Can you work these out from the model? Positions are in its coordinate system, mm. A direction names the side the tool comes from. Give positions to 0.01 mm unless a question says otherwise; leave off trailing zeros. Order: outer loops, then holes, each group sorted by start corner. A loop starts at its lowest first (then second) coordinate and runs counter-clockwise, first axis right, second up. Notation, with made-up numbers: (3, -17) - (29, -17) arc R18 cw to (29, -10) - close; hole circle Ø3 at (-33.75, 59.5). An arc over 180 degrees is marked (long way). Return JSON: item names as keys, results as strings.
```python
from build123d import *

# Parameters (mm, degrees)
SALIENTE_EXTRUIR1_DEPTH = 20
CORTAR_EXTRUIR1_REACH   = 24.289
CROQUIS2_R              = 3.75
SALIENTE_EXTRUIR2_START = -9
CROQUIS3_R              = 3.75
SALIENTE_EXTRUIR2_DEPTH = 9
CROQUIS4_R              = 4.765
SALIENTE_EXTRUIR3_DEPTH = 70
CROQUIS5_R              = 13.287682266
SALIENTE_EXTRUIR4_DEPTH = 4.5


with BuildPart() as part:
    # Croquis1 → Saliente-Extruir1 (new body)
    with BuildSketch(Plane.XY):
        Polygon((-8.75, 2.25), (8.75, 2.25), (4.25, -2.25), (-4.25, -2.25), align=None)
    extrude(amount=SALIENTE_EXTRUIR1_DEPTH)

    # Croquis2 → Cortar-Extruir1 (cut, up to next)
    with BuildSketch(Plane(origin=(0, 2.25, 0), x_dir=(1, 0, 0), z_dir=(0, 1, 0)), mode=Mode.PRIVATE) as cortar_extruir1_sk1:
        with Locations(Location((0, -10, 0), (0, 0, 270))):
            Circle(CROQUIS2_R)
    cortar_extruir1_tool1 = extrude(cortar_extruir1_sk1.sketch, amount=-CORTAR_EXTRUIR1_REACH, mode=Mode.PRIVATE) & part.part
    add(cortar_extruir1_tool1.solids().sort_by_distance((0, 2.25, 10))[0], mode=Mode.SUBTRACT)

    # Croquis3 → Saliente-Extruir2 (add)
    with BuildSketch(Plane.XZ.offset(2.25).offset(SALIENTE_EXTRUIR2_START)):
        with Locations(Location((0, 10, 0), (0, 0, 270))):
            Circle(CROQUIS3_R)
    extrude(amount=SALIENTE_EXTRUIR2_DEPTH)

    # Croquis4 → Saliente-Extruir3 (add)
    with BuildSketch(Plane(origin=(0, 6.75, 0), x_dir=(1, 0, 0), z_dir=(0, 1, 0))):
        with Locations(Location((0, -10, 0), (0, 0, 270))):
            Circle(CROQUIS4_R)
    extrude(amount=SALIENTE_EXTRUIR3_DEPTH)

    # Croquis5 → Saliente-Extruir4 (add)
    with BuildSketch(Plane(origin=(0, 2.25, 0), x_dir=(1, 0, 0), z_dir=(0, 1, 0))):
        with Locations(Location((0, -10, 0), (0, 0, 270))):
            Circle(CROQUIS5_R)
    extrude(amount=-SALIENTE_EXTRUIR4_DEPTH)


solid = part.part
```
1. Suppose I cut it at C-C (y = 35.5). List the corners of the cut face in (x, z) for me (3 decimals), plus the area to 3 significant figures.
Checks:
{"outline": "circle Ø9.53 at (0, 10)", "area": "71.3 mm^2"}
2. If I drill on L1, parallel to Y at x = 2.25, z = 13.5; L2, parallel to Y at x = -4.25, z = 2.75; L3, parallel to X at y = 29, z = 10 (3 decimals), over which ranges is the centre line in solid material (lowest first)? Write a range as [from, to].
Checks:
{"L1": "[-2.25, 2.25], [6.75, 76.75]", "L2": "[-2.25, 2.25]", "L3": "[-4.765, 4.765]"}
3. Suppose I cut it at B-B (z = 10). List the corners of the cut face in (x, y) for me (3 decimals), plus the area to 3 significant figures.
Checks:
{"outline": "(-13.288, -2.25) - (13.288, -2.25) - (13.288, 2.25) - (3.75, 2.25) - (3.75, 6.75) - (4.765, 6.75) - (4.765, 76.75) - (-4.765, 76.75) - (-4.765, 6.75) - (-3.75, 6.75) - (-3.75, 2.25) - (-13.288, 2.25) - close", "area": "820 mm^2"}
4. Suppose I cut it at A-A (x = 0). List the corners of the cut face in (y, z) for me (3 decimals).
Checks:
{"outline": "(-2.25, -3.288) - (2.25, -3.288) - (2.25, 6.25) - (6.75, 6.25) - (6.75, 5.235) - (76.75, 5.235) - (76.75, 14.765) - (6.75, 14.765) - (6.75, 13.75) - (2.25, 13.75) - (2.25, 23.288) - (-2.25, 23.288) - close"}
5. Suppose I cut it at D-D (z = 20.25). List the corners of the cut face in (x, y) for me.
Checks:
{"outline": "(-8.46, -2.25) - (8.46, -2.25) - (8.46, 2.25) - (-8.46, 2.25) - close"}
6. On a 3-axis mill with a long thin cutter (end or side, diameter ignored), from which of +Z, -Z, +X, -X, +Y, -Y can I reach the whole of each face in a straight line? I mean faces 4 (the face through (0.584, 0.031, -3.275)), 5 (the face through (-1, 6.75, 6)). Say none if no direction works.
Checks:
{"face 4": "+Y, -Y", "face 5": "none"}
7. For pin 1 Ø2 at (y, z) = (44, 3.5) entering from +X; pin 2 Ø5 at (y, z) = (33, 14) entering from +X; pin 3 Ø4 at (y, z) = (28, 14) entering from -X; pin 4 Ø8 at (y, z) = (41.5, 12.5) entering from -X (3 decimals), each with a flat end and sliding along its axis, tell me the tip position at first contact or that it passes through.
Checks:
{"pin 1": "through", "pin 2": "x = 4.52", "pin 3": "x = -4.32", "pin 4": "x = -4.765"}
8. Thinking about a two-plate mould opening in Y: for faces 1 (the face through (0.165, 4.531, 13.746)), 2 (the face through (0, 76.75, 10)), 3 (the face through (0.21, 41.26, 5.24)), which applies, +Y half, -Y half, draft (parallel to the pull), parting line (faces both ways), or undercut?
Checks:
{"face 1": "undercut", "face 2": "+Y half", "face 3": "draft"}
